CAD build for the part. Positions are in the model's coordinates, mm. Face numbers are marked on the shaded views. Give positions to 0.01 mm unless a question says otherwise; leave off trailing zeros. Loops run counter-clockwise (first coordinate to the right, second up) from the corner with the lowest first, then second, coordinate; pieces in that order, holes last.
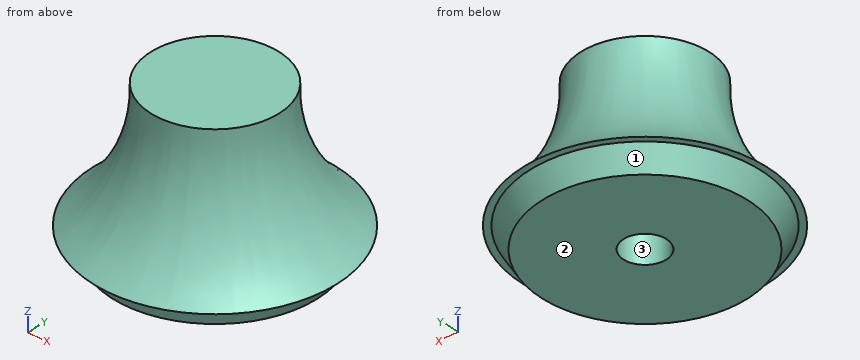
```python
from build123d import *

# Parameters (mm, degrees)
F2_R     = 5
F3_DEPTH = 32


with BuildPart() as f1:
    # F0 (on Front) → F1 (revolve)
    with BuildSketch(Plane.XZ):
        with BuildLine():
            Line((0, 35), (0, 0))
            Line((0, 0), (24, 0))
            Line((24, 0), (27, 5))
            Line((27, 5), (28.5, 5))
            ThreePointArc((28.5, 5), (18.243075, 18.421884), (15, 35))
            Line((15, 35), (0, 35))
        make_face()
    revolve(axis=Axis((0, 0, 17.5), (0, 0, -1)))


with BuildPart() as f3:
    # F2 (on Top) → F3 (new body)
    with BuildSketch(Plane.XY):
        Circle(F2_R)
    extrude(amount=F3_DEPTH)


with BuildPart() as f1_1:
    add(f1.part)

    # F4: cut F3
    add(f3.part, mode=Mode.SUBTRACT)


solid = f1_1.part
```
1. Drop flat-ended pins along their axis: pin 1 (6 mm diameter, centred on x = 2.5, z = 30, fed in from -Y); pin 2 (6 mm diameter, centred on x = -1.5, y = 0.5, fed in from -Z); pin 3 (6 mm diameter, centred on x = -13.5, y = -11, fed in from +Z); pin 4 (10 mm diameter, centred on x = 21.5, z = 11, fed in from -Y). Give the stop position or say it passes through.
Responses:
pin 1: stops at y = -15.48
pin 2: stops at z = 32
pin 3: stops at z = 35
pin 4: stops at y = -18.65
2. Probe line 1 along Y through (x, z) = (0, 10); line 2 along Y through (x, z) = (0, 21); line 3 along Z through (x, y) = (-20, 14.5). List the from-to ranges inside material, lowest first.
Responses:
line 1: y = -23.49 to -5, 5 to 23.49
line 2: y = -17.2 to -5, 5 to 17.2
line 3: z = 1.17 to 8.6
3. Saw through at D-D, the plane z = 33.5. List the corners of the cut face in (x, y).
Responses:
outline: circle Ø29.95 at (0, 0)
4. Saw through at A-A, the plane y = 0. List the corners of the cut face in (x, z).
Responses:
outline: (-28.5, 5) - (-27, 5) - (-24, 0) - (-5, 0) - (-5, 32) - (5, 32) - (5, 0) - (24, 0) - (27, 5) - (28.5, 5) arc R37.1 cw to (15, 35) - (-15, 35) arc R37.1 cw to start
5. Saw through at C-C, the plane z = 21. List the corners of the cut face in (x, y).
Responses:
outline: circle Ø34.39 at (0, 0); hole circle Ø10 at (0, 0)
6. Pull direction X, two halves, no side cores. Call the marked faces 1, 2 and 3: released by +X, released by -X, zero draft, split by the parting line, or undercut.
Responses:
face 1: split by the parting line
face 2: zero draft
face 3: undercut
